Model file for the job. Use its own axes, mm. Face numbers are marked on the shaded views. A direction names the side the tool comes from. Round coordinates to 2 decimals unless told otherwise and drop trailing zeros. Order: outer loops, then holes, each group sorted by start corner. A loop starts at its lowest first (then second) coordinate and runs counter-clockwise, first axis right, second up. Notation, with made-up numbers: (25, 1.25) -> (33, 1.25) arc R18 cw to (33, 8.25) -> close; hole circle Ø10 at (-11, -12). An arc over 180 degrees is marked (long way). Answer as CSV lines item,"result".
Autodesk Fusion 360 part; units mm, degrees
sketch "Sketch1" plane through (0, 0, 0) normal (1, 0, 0) x (0, 1, 0)
  circle A0 centre (0, 0) radius 35
  dimension "d1" = 70
extrude "Extrude1" add sketch "Sketch1" along normal blind 10 in component "Encaixe"
sketch "Sketch3" plane through (10, 0, 0) normal (1, 0, 0) x (0, 1, 0)
  circle A0 centre (0, 0) radius 35
  circle A1 centre (0, 0) radius 23.5
  dimension "d9" = 47
extrude "Extrude2" add sketch "Sketch3" along normal blind 13 contours A1 in component "Encaixe"
ref_plane "WorkPlane1" through (0, 13, 0) normal (0, 1, 0) x (0, 0, 1)
sketch "Sketch4" plane through (0, 13, 0) normal (0, 1, 0) x (1, 0, 0)
  line L0 (23, 0) -> (23, -35)
  line L1 (23, -35) -> (23, -45)
  line L2 (23, -35) -> (30.3921, -43.8095)
  line L3 (30.3921, -43.8095) -> (35.3921, -43.8095)
  line L4 (23, 0) -> (57, 0)
  line L5 (35.3921, -43.8095) -> (52.4338, -23.5)
  line L6 (35.3921, -43.8095) -> (44, -43.8095)
  line L7 (52.4338, -23.5) -> (52.4338, 0)
  line L8 (52.4338, 23.5) -> (52.4338, 0)
  line L9 (35.3921, 43.8095) -> (52.4338, 23.5)
  line L10 (30.3921, 43.8095) -> (35.3921, 43.8095)
  line L11 (23, 35) -> (30.3921, 43.8095)
  line L12 (23, 0) -> (23, 35)
  dimension "d13" = 35
  dimension "d14" = 10
  dimension "d15" = 11.5
  dimension "d16" = 40
  dimension "d17" = 5
  dimension "d18" = 50
sketch "Sketch10" plane through (23, 0, 0) normal (1, 0, 0) x (0, 1, 0)
  circle A0 centre (0, 0) radius 23.5
  line L0 (0, 0) -> (18.3161, -14.7232) construction
  line L1 (0, 0) -> (18.3161, 14.7232) construction
  line L2 (0, 0) -> (-18.3161, 14.7232) construction
  line L3 (0, 0) -> (-18.3161, -14.7232) construction
  arc A1 (18.3161, -14.7232) -> (18.3161, 14.7232) centre (0, 0) ccw construction
  arc A2 (-18.3161, 14.7232) -> (-18.3161, -14.7232) centre (0, 0) ccw construction
  line L4 (0, 0) -> (-23.5, 0) construction
  line L5 (-23.5, 0) -> (-18, 0)
  line L6 (-18, 0) -> (-18, 7) construction
  circle A3 centre (-18, 7) radius 3
  circle A4 centre (-18, -7) radius 3
  line L7 (0, 0) -> (0, 10) construction
  circle A5 centre (18, 7) radius 3
  circle A6 centre (18, -7) radius 3
  dimension "d43" = 102.413
  dimension "d45" = 6
extrude "Extrude8" cut sketch "Sketch10" against normal blind 10 contours A3 | A4 | A5 | A6 in component "Encaixe"
thread "Thread1" in component "Encaixe"
thread "Thread2" in component "Encaixe"
thread "Thread3" in component "Encaixe"
thread "Thread4" in component "Encaixe"
sketch "Sketch11" plane through (0, 0, 0) normal (-1, 0, 0) x (0, -1, 0)
  circle A0 centre (0, 0) radius 35
  circle A1 centre (0, 0) radius 10
  dimension "d48" = 20
extrude "Extrude9" cut sketch "Sketch11" against normal blind 10 contours A1 in component "Encaixe"
extrude "Extrude10" cut 1 faces at (10, -3.1852, -0.9825) along direction (1, 0, 0) blind 5 in component "Encaixe"
sketch "Sketch12" plane through (15, 0, 0) normal (-1, 0, 0) x (0, -1, 0)
  circle A0 centre (0, 0) radius 10
  line L0 (3, 3) -> (3, 9.5394)
  line L1 (-3, 3) -> (-3, 9.5394)
  line L2 (-3, -3) -> (-9.5394, -3)
  line L3 (-3, 3) -> (-9.5394, 3)
  line L4 (3, -3) -> (3, -9.5394)
  line L5 (-3, -3) -> (-3, -9.5394)
  line L6 (3, 3) -> (9.5394, 3)
  line L7 (3, -3) -> (9.5394, -3)
extrude "Extrude11" add sketch "Sketch12" along normal blind 15 contours A0 L0 L6 | A0 L4 L7 | A0 L1 L3 | A0 L2 L5 in component "Encaixe"
component "Encaixe" placed x (1, 0, 0) y (0, 1, 0) z (0, 0, 1) at (0, 0, 0)
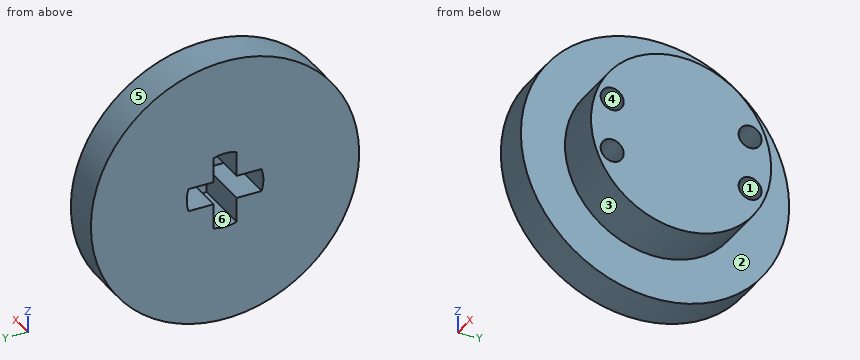
Q1. Saw through at B-B (x = 2). Write the cut outline in (y, z).
Checks:
outline,"circle Ø70 at (0, 0); hole (-9.54, -3) -> (-3, -3) -> (-3, -9.54) arc R10 ccw to (3, -9.54) -> (3, -3) -> (9.54, -3) arc R10 ccw to (9.54, 3) -> (3, 3) -> (3, 9.54) arc R10 ccw to (-3, 9.54) -> (-3, 3) -> (-9.54, 3) arc R10 ccw to start"
Q2. Saw through at D-D (y = 18). Write the cut outline in (x, z), plus the area to 3 significant figures.
Checks:
outline,"(0, -30.02) -> (10, -30.02) -> (10, -15.11) -> (23, -15.11) -> (23, -10) -> (13, -10) -> (13, -4) -> (23, -4) -> (23, 4) -> (13, 4) -> (13, 10) -> (23, 10) -> (23, 15.11) -> (10, 15.11) -> (10, 30.02) -> (0, 30.02) -> close"
area,"873 mm²"
Q3. Saw through at C-C (z = 0). Write the cut outline in (x, y), plus the area to 3 significant figures.
Checks:
outline,"(0, -35) -> (10, -35) -> (10, -23.5) -> (23, -23.5) -> (23, 23.5) -> (10, 23.5) -> (10, 35) -> (0, 35) -> (0, 10) -> (15, 10) -> (15, -10) -> (0, -10) -> close"
area,"1,010 mm²"
Q4. Saw through at A-A (x = 16.25). Write the cut outline in (y, z), plus the area to 3 significant figures.
Checks:
outline,"circle Ø47 at (0, 0); hole circle Ø6 at (-18, -7); hole circle Ø6 at (-18, 7); hole circle Ø6 at (18, -7); hole circle Ø6 at (18, 7)"
area,"1,620 mm²"
Q5. Flat gauge pins, fed straight in: pin 1 (3.5 mm diameter, centred on x = 9.5, z = -5.5, fed in from -Y); pin 2 (3 mm diameter, centred on y = -18.5, z = 7.5, fed in from +X); pin 3 (7 mm diameter, centred on x = 4.5, z = 6.5, fed in from +Y). Where does each tip first touch, or does it go through?
Checks:
pin 1,"y = -34.8"
pin 2,"x = 13"
pin 3,"y = 34.87"
Q6. Wall check: L1, parallel to Y at x = 13.25, z = 0.5; L2, parallel to Z at x = 15.5, y = -18; L3, parallel to X at y = 5, z = -23.5. Give the ranges that are in metal, low to high. Write a range as [from, to].
Checks:
L1,"[-23.49, -9.99], [9.99, 23.49]"
L2,"[-15.11, -10], [-4, 4], [10, 15.11]"
L3,"[0, 10]"
Q7. Mould opens along Z. For the marked faces 1, 2 and 3 say: +Z half, -Z half, draft (parallel to the pull), parting line (faces both ways), or undercut.
Checks:
face 1,"undercut"
face 2,"draft"
face 3,"parting line"
Q8. Tool access for the marked faces 4, 5 and 6: list every direction of +Z, -Z, +X, -X, +Y, -Y with a clear straight run to the whole face (end or side of a thin tool).
Checks:
face 4,"+X"
face 5,"+X, -X"
face 6,"-X"
